Input: part model. Units: mm. Frame: model coordinates. A direction names the side the tool comes from. Coordinates: 2 decimals unless noted, no trailing zeros. Write each loop counter-clockwise with the first axis right and the second up, starting at its lowest first coordinate (ties: lowest second). Pieces come first, ordered by that corner, then holes. Notation, with made-up numbers: M -27,-7 L -11,-7 A19 cw -11,21 Z; hole C 5.5,1.5 d7. An arc over 180 degrees is marked long. Use one line per item in the form item = value.
from build123d import *

# Parameters (mm, degrees)
F0_R     = 2.5
F1_DEPTH = 145
F3_DEPTH = 5
F5_DEPTH = 5
F7_DEPTH = 5


with BuildPart() as f1:
    # F0 (on Top) → F1 (new body)
    with BuildSketch(Plane.XY):
        Circle(F0_R)
    extrude(amount=F1_DEPTH)

    # F2 (on face) → F3 (join)
    with BuildSketch(Plane.XY.offset(145)):
        with BuildLine():
            Line((2.5, 2.5), (0, 2.5))
            ThreePointArc((0, 2.5), (1.767766953, 1.767766953), (2.5, 0))
            Line((2.5, 0), (2.5, 2.5))
        make_face()
        with BuildLine():
            Line((2.5, -2.5), (2.5, 0))
            ThreePointArc((2.5, 0), (1.767766953, -1.767766953), (0, -2.5))
            Line((0, -2.5), (2.5, -2.5))
        make_face()
        with BuildLine():
            ThreePointArc((2.5, 0), (1.767766953, 1.767766953), (0, 2.5))
            ThreePointArc((0, 2.5), (-1.767766953, 1.767766953), (-2.5, 0))
            ThreePointArc((-2.5, 0), (-1.767766953, -1.767766953), (0, -2.5))
            ThreePointArc((0, -2.5), (1.767766953, -1.767766953), (2.5, 0))
        make_face()
        with BuildLine():
            Line((0, 2.5), (-2.5, 2.5))
            Line((-2.5, 2.5), (-2.5, 0))
            ThreePointArc((-2.5, 0), (-1.767766953, 1.767766953), (0, 2.5))
        make_face()
        with BuildLine():
            ThreePointArc((0, -2.5), (-1.767766953, -1.767766953), (-2.5, 0))
            Line((-2.5, 0), (-2.5, -2.5))
            Line((-2.5, -2.5), (0, -2.5))
        make_face()
    extrude(amount=F3_DEPTH)

    # F4 (on face) → F5 (join)
    with BuildSketch(Plane(origin=(-2.5, 0, 0), x_dir=(0, -1, 0), z_dir=(-1, 0, 0))):
        with BuildLine():
            ThreePointArc((-2.5, 147.5), (-1.767766953, 145.732233047), (0, 145))
            ThreePointArc((0, 145), (1.767766953, 145.732233047), (2.5, 147.5))
            ThreePointArc((2.5, 147.5), (1.767766953, 149.267766953), (0, 150))
            ThreePointArc((0, 150), (-1.767766953, 149.267766953), (-2.5, 147.5))
        make_face()
    extrude(amount=F5_DEPTH)

    # F6 (on face) → F7 (join)
    with BuildSketch(Plane.YZ.offset(2.5)):
        with BuildLine():
            ThreePointArc((-2.5, 147.5), (-1.767766953, 145.732233047), (0, 145))
            ThreePointArc((0, 145), (1.767766953, 145.732233047), (2.5, 147.5))
            ThreePointArc((2.5, 147.5), (1.767766953, 149.267766953), (0, 150))
            ThreePointArc((0, 150), (-1.767766953, 149.267766953), (-2.5, 147.5))
        make_face()
    extrude(amount=F7_DEPTH)


solid = f1.part
(1) Section query A-A on y = 1.1. Return the cut outline in (x, z) (3 decimals).
Computed:
outline = M -7.5,145.255 L -2.5,145.255 L -2.5,145 L -2.245,145 L -2.245,0 L 2.245,0 L 2.245,145 L 2.5,145 L 2.5,145.255 L 7.5,145.255 L 7.5,149.745 L 2.5,149.745 L 2.5,150 L -2.5,150 L -2.5,149.745 L -7.5,149.745 Z
(2) Line query: probe 1 along Z at (x, y) = (-1.5, -2.1); probe 2 along X at (y, z) = (0.1, 17.5); probe 3 along Z at (x, y) = (5.25, -1.2). Output: solid intervals per line, ascending.
Computed:
probe_1 = 145 to 150
probe_2 = -2.5 to 2.5
probe_3 = 145.31 to 149.69
(3) Section query B-B on x = -4.25. Return the cut outline in (y, z), plus the area to 3 significant figures.
Computed:
outline = C 0,147.5 d5
area = 19.6 mm^2
(4) First-contact query: pin 1 Ø2 at (x, z) = (-1.5, 122.5) entering from -Y; pin 2 Ø2.5 at (x, y) = (-1, -1) entering from -Z; pin 3 Ø2 at (x, z) = (-2, 37.5) entering from +Y; pin 4 Ø1 at (x, z) = (2, 119) entering from -Y. Flat tips, straight axial feed; report the tip coordinate or a pass-through.
Computed:
pin_1 = -2.45
pin_2 = 0
pin_3 = 2.29
pin_4 = -2
(5) Section query C-C on z = 127. Return the cut outline in (x, y).
Computed:
outline = C 0,0 d5
(6) Set-up query: faces 1 (the flat face through (2.5, -2, 149.4)), 2 (the flat face through (2, -2, 145)), 3 (the flat face through (-2.5, 2, 145.6)), 4 (the flat face through (-2, -2, 145)). Return all of +Z, -Z, +X, -X, +Y, -Y with unobstructed straight access to the full face (end or side cutting, diameter ignored); none if empty.
Computed:
face_1 = +Z, +X, -Y
face_2 = -Z, +X, -Y
face_3 = -Z, -X, +Y
face_4 = -Z, -X, -Y
